Can you work these out from the model? Positions are in its coordinate system, mm. A direction names the side the tool comes from. Round coordinates to 2 decimals unless told otherwise and drop trailing zeros. Loops run counter-clockwise (first coordinate to the right, second up) from the corner with the lowest first, then second, coordinate; pieces in that order, holes last. Notation, with made-up numbers: M -2.5,-39 L 31.5,-39 A33 cw 31.5,-3 Z; hole C 15.5,26.25 d8. An arc over 180 degrees is marked long. Answer as CSV lines item,"result".
from build123d import *

# Parameters (mm, degrees)
SKETCH1_R           = 1.7
BOSS_EXTRUDE1_DEPTH = 2
SKETCH2_W           = 2
SKETCH2_H           = 2
BOSS_EXTRUDE2_DEPTH = 126
SKETCH3_R           = 1.7
BOSS_EXTRUDE3_DEPTH = 2
CHAMFER1_SIZE       = 0.7


with BuildPart() as part:
    # Sketch1 → Boss-Extrude1 (new body)
    with BuildSketch(Plane.XY):
        with BuildLine():
            Line((0, 0), (0, 10))
            ThreePointArc((0, 10), (7.071067812, 7.071067812), (10, 0))
            Line((10, 0), (0, 0))
        make_face()
        with Locations((5, 5)):
            Circle(SKETCH1_R, mode=Mode.SUBTRACT)
    extrude(amount=BOSS_EXTRUDE1_DEPTH)

    # Sketch2 → Boss-Extrude2 (add)
    with BuildSketch(Plane.XY.offset(2)):
        with Locations((1, 1)):
            Rectangle(SKETCH2_W, SKETCH2_H)
        with BuildLine():
            Line((0, 10), (0, 2))
            Line((0, 2), (2, 2))
            Line((2, 2), (2, 9.797958971))
            ThreePointArc((2, 9.797958971), (1.00508962, 9.94936153), (0, 10))
        make_face()
        with BuildLine():
            Line((2, 2), (2, 0))
            Line((2, 0), (10, 0))
            ThreePointArc((10, 0), (9.94936153, 1.00508962), (9.797958971, 2))
            Line((9.797958971, 2), (2, 2))
        make_face()
    extrude(amount=BOSS_EXTRUDE2_DEPTH)

    # Sketch3 → Boss-Extrude3 (add)
    # profile 1 of 2: a face of its own
    with BuildSketch(Plane.XY.offset(128)):
        with BuildLine():
            ThreePointArc((9.797958971, 2), (7.071067812, 7.071067812), (2, 9.797958971))
            Line((2, 9.797958971), (2, 2))
            Line((2, 2), (9.797958971, 2))
        make_face()
        with Locations((5, 5)):
            Circle(SKETCH3_R, mode=Mode.SUBTRACT)
    # profile 2 of 2: a face of its own
    with BuildSketch(Plane.XY.offset(128)):
        with BuildLine():
            ThreePointArc((10, 0), (9.94936153, 1.00508962), (9.797958971, 2))
            Line((9.797958971, 2), (2, 2))
            Line((2, 2), (2, 9.797958971))
            ThreePointArc((2, 9.797958971), (1.00508962, 9.94936153), (0, 10))
            Line((0, 10), (0, 0))
            Line((0, 0), (10, 0))
        make_face()
    extrude(amount=BOSS_EXTRUDE3_DEPTH)

    # Chamfer1
    # the kernel refuses this chamfer: 0.7 mm, written as the material it adds along each edge
    with BuildSketch(Plane(origin=(11.598137063, 2, 128), x_dir=(0, -0.027495876610586324, -0.9996219169112966), z_dir=(-1, 0, 0))) as chamfer1_piece_1_section:
        Polygon((CHAMFER1_SIZE * 0.999621916911, -CHAMFER1_SIZE * 0.0274958766106), (-CHAMFER1_SIZE * 0.0274958766106, -CHAMFER1_SIZE * 0.999621916911), (0, 0), align=None)
    chamfer1_piece_1 = extrude(amount=11.398315154, mode=Mode.PRIVATE)
    chamfer1_piece_1 = chamfer1_piece_1 & Plane(origin=(0, 0, 127.768642056), x_dir=(0, 1, 0), z_dir=(0, 0, -1)) * Cylinder(10, 26, mode=Mode.PRIVATE)
    add(chamfer1_piece_1)
    with BuildSketch(Plane(origin=(2, 11.598137063, 2), x_dir=(0.9996219169112968, 0, -0.027495876610586445), z_dir=(0, -1, 0))) as chamfer1_piece_2_section:
        Polygon((CHAMFER1_SIZE * 0.999621916911, CHAMFER1_SIZE * 0.0274958766106), (-CHAMFER1_SIZE * 0.0274958766106, CHAMFER1_SIZE * 0.999621916911), (0, 0), align=None)
    chamfer1_piece_2 = extrude(amount=11.398315154, mode=Mode.PRIVATE)
    chamfer1_piece_2 = chamfer1_piece_2 & Plane(origin=(0, 0, 2.231357944), x_dir=(0, 1, 0), z_dir=(0, 0, -1)) * Cylinder(10, 26, mode=Mode.PRIVATE)
    add(chamfer1_piece_2)
    with BuildSketch(Plane(origin=(2, 0.199821908, 128), x_dir=(0.9996219169112962, 0, 0.027495876610605856), z_dir=(0, 1, 0))) as chamfer1_piece_3_section:
        Polygon((CHAMFER1_SIZE * 0.999621916911, CHAMFER1_SIZE * 0.0274958766106), (-CHAMFER1_SIZE * 0.0274958766106, CHAMFER1_SIZE * 0.999621916911), (0, 0), align=None)
    chamfer1_piece_3 = extrude(amount=11.398315154, mode=Mode.PRIVATE)
    chamfer1_piece_3 = chamfer1_piece_3 & Plane(origin=(0, 0, 127.769144461), x_dir=(0, 1, 0), z_dir=(0, 0, -1)) * Cylinder(10, 26, mode=Mode.PRIVATE)
    add(chamfer1_piece_3)
    with BuildSketch(Plane(origin=(11.598137063, 2, 2), x_dir=(0, 0.9996219169112968, -0.027495876610586445), z_dir=(-1, 0, 0))) as chamfer1_piece_4_section:
        Polygon((CHAMFER1_SIZE * 0.999621916911, -CHAMFER1_SIZE * 0.0274958766106), (-CHAMFER1_SIZE * 0.0274958766106, -CHAMFER1_SIZE * 0.999621916911), (0, 0), align=None)
    chamfer1_piece_4 = extrude(amount=11.398315154, mode=Mode.PRIVATE)
    chamfer1_piece_4 = chamfer1_piece_4 & Plane(origin=(0, 0, 2.231357944), x_dir=(0, 1, 0), z_dir=(0, 0, -1)) * Cylinder(10, 26, mode=Mode.PRIVATE)
    add(chamfer1_piece_4)


solid = part.part
Item 1: On a 3-axis mill with a long thin cutter (end or side, diameter ignored), from which of +Z, -Z, +X, -X, +Y, -Y can I reach the whole of each face in a straight line? I mean faces 5 (the face through (7, 5, 128)), 6 (the face through (5, 0, 64)). Say none if no direction works.
Output:
face 5,"+X, +Y"
face 6,"+Z, -Z, +X, -X, -Y"
Item 2: If we section it at A-A on x = 5: Write out the boundary of the cut face in (y, z), then the cut area to 3 significant figures.
Output:
outline,"M 0,0 L 3.3,0 L 3.3,2 L 2.7,2 L 2,2.7 L 2,127.3 L 2.7,128 L 3.3,128 L 3.3,130 L 0,130 Z; M 6.7,0 L 8.66,0 L 8.66,2 L 6.7,2 Z; M 6.7,128 L 8.66,128 L 8.66,130 L 6.7,130 Z"
area,"274 mm2"
Item 3: We'd pull the mould along X, two halves only. Please class faces 1 (the face through (0, 5, 64)), 2 (the face through (5.8, 3.5, 1)), 3 (the face through (5, 7, 2)), 4 (the face through (5.8, 3.5, 129)): released by +X, released by -X, zero draft, split by the parting line, or undercut.
Output:
face 1,"released by -X"
face 2,"undercut"
face 3,"zero draft"
face 4,"undercut"
Item 4: Will these pins go through, and if not, where does the flat tip stop? pin 1 (1.5 mm diameter, centred on y = 5.5, z = 47.5, fed in from +X); pin 2 (2.5 mm diameter, centred on x = 5, z = 53, fed in from +Y).
Output:
pin 1,"stops at x = 2"
pin 2,"stops at y = 2"
Item 5: If I drill on line 1 along Z through (x, y) = (3, 5); line 2 along Y through (x, z) = (5.75, 46), over which ranges is the centre line in solid material (lowest first)? Write a range as from..to.
Output:
line 1,"z = 0..2, 128..130"
line 2,"y = 0..2"
Item 6: If we section it at C-C on z = 108: Write out the boundary of the cut face in (x, y).
Output:
outline,"M 0,0 L 10,0 A10 ccw 9.8,2 L 2,2 L 2,9.8 A10 ccw 0,10 Z"
